Could you check a few things on this drawing? It's one solid part, dimensions in mm from its lowest x, y, z. Round coordinates to 2 decimals unless told otherwise and drop trailing zeros. Write each loop counter-clockwise with the first axis right and the second up, starting at its lowest first coordinate (ties: lowest second). Pieces come first, ordered by that corner, then holes. Notation, with made-up numbers: M 76,-5.5 L 112,-5.5 A36 ccw 112,32.5 Z; hole C -29,-27 d6. An arc over 180 degrees is marked long. One line per item, written item: value. Start each with the question number.
(1) I want a section at D-D on x = 252. Please give me the cut outline in (y, z).
(2) If I drill on L1, parallel to Y at x = 139.7, z = 2.2 (1 decimal); L2, parallel to Y at x = 142, z = 3.65, over which ranges is the centre line in solid material (lowest first)?
(3) I want a section at B-B on x = 139.7. Please give me the cut outline in (y, z) (1 decimal), and give its area (3 significant figures).
(4) I'm going to push flat-ended pins straight in: pin 1 Ø12 at (x, y) = (39, 62.5) entering from -Z; pin 2 Ø1 at (y, z) = (42.5, 0.5) entering from -X; pin 3 Ø3 at (x, z) = (78, 1.5) entering from -Y; pin 4 Ø1 at (x, z) = (59, 4) entering from +Y. Where does each tip first touch, or does it pass through?
(5) I want a section at A-A on z = 3. Please give me the cut outline in (x, y) (1 decimal).
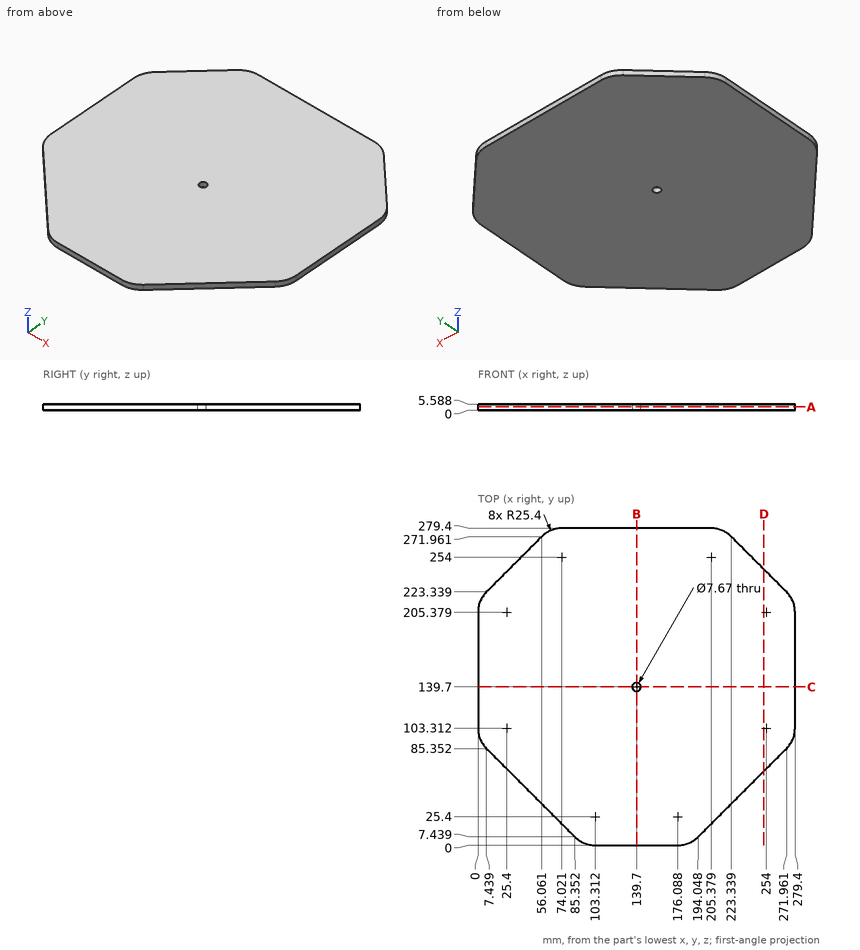
Found:
1. outline: M 65.39,0 L 243.3,0 L 243.3,5.59 L 65.39,5.59 Z
2. L1: y = 0 to 135.9, 143.5 to 279.4
2. L2: y = 0 to 136.63, 142.77 to 279.4
3. outline: M 0,0 L 135.9,0 L 135.9,5.6 L 0,5.6 Z; M 143.5,0 L 279.4,0 L 279.4,5.6 L 143.5,5.6 Z
3. area: 1,520 mm²
4. pin 1: stops at z = 0
4. pin 2: stops at x = 49.79
4. pin 3: stops at y = 13.29
4. pin 4: stops at y = 274.84
5. outline: M 0,103.3 A25.4 ccw 7.4,85.4 L 85.4,7.4 A25.4 ccw 103.3,0 L 176.1,0 A25.4 ccw 194,7.4 L 272,85.4 A25.4 ccw 279.4,103.3 L 279.4,205.4 A25.4 ccw 272,223.3 L 223.3,272 A25.4 ccw 205.4,279.4 L 74,279.4 A25.4 ccw 56.1,272 L 7.4,223.3 A25.4 ccw 0,205.4 Z; hole C 139.7,139.7 d7.7
